```python
from build123d import *

# Parameters (mm, degrees)
ESQUISSE1_W             = 32
ESQUISSE1_H             = 8
BOSS_EXTRU_1_DEPTH      = 2
BOSS_EXTRU_2_DEPTH      = 2
ESQUISSE3_R             = 1.9999999999999996
ESQUISSE3_R_2           = 2.000000000000003
ESQUISSE3_R_3           = 1.9999999999999991
BOSS_EXTRU_3_DEPTH      = 2
ESQUISSE4_R             = 1.2499999999999991
ESQUISSE4_R_2           = 1.250000000000001
ESQUISSE4_R_3           = 1.2500000000000013
ENL_V_MAT_EXTRU_1_DEPTH = 2
CONG_1_R                = 1.5


with BuildPart() as part:
    # Esquisse1 → Boss.-Extru.1 (new body)
    with BuildSketch(Plane(origin=(0, 0, 0), x_dir=(1, 0, 0), z_dir=(0, 1, 0))):
        with Locations((16, 4)):
            Rectangle(ESQUISSE1_W, ESQUISSE1_H)
    extrude(amount=BOSS_EXTRU_1_DEPTH)

    # Esquisse2 → Boss.-Extru.2 (add)
    with BuildSketch(Plane(origin=(0, 2, 0), x_dir=(1, 0, 0), z_dir=(0, 1, 0))):
        Polygon((8.000000000000002, 4.5e-16), (24, 2.41e-15), (24.000000000000004, -17), (8.000000000000004, -17), align=None)
    extrude(amount=-BOSS_EXTRU_2_DEPTH)

    # Esquisse3 → Boss.-Extru.3 (add)
    with BuildSketch(Plane(origin=(0, 2, 0), x_dir=(1, 0, 0), z_dir=(0, 1, 0))):
        with Locations((8.000000000000002, 0)):
            Circle(ESQUISSE3_R)
        with Locations((24, 2.41e-15)):
            Circle(ESQUISSE3_R_2)
        with Locations((16.000000000000004, -17)):
            Circle(ESQUISSE3_R_3)
    extrude(amount=-BOSS_EXTRU_3_DEPTH)

    # Esquisse4 → Enlèv. mat.-Extru.1 (cut)
    with BuildSketch(Plane(origin=(0, 2, 0), x_dir=(1, 0, 0), z_dir=(0, 1, 0))):
        with Locations(Location((8.000000000000002, 0, 0), (0, 0, 270))):
            Circle(ESQUISSE4_R)
        with Locations(Location((24, 2.41e-15, 0), (0, 0, 270))):
            Circle(ESQUISSE4_R_2)
        with Locations(Location((16.000000000000004, -17, 0), (0, 0, 270))):
            Circle(ESQUISSE4_R_3)
    extrude(amount=-ENL_V_MAT_EXTRU_1_DEPTH, mode=Mode.SUBTRACT)

    # Congé1
    cong_1_edges = [part.edges().sort_by_distance(p)[0] for p in [
        (32, 2, -4),
        (16, 2, -8),
        (11.000000000000004, 2, 17),
        (24.000000000000004, 2, 9.500000000000002),
        (8.000000000000004, 2, 9.5),
        (29, 2, 0),
        (0, 2, -4),
        (21.000000000000004, 2, 17),
        (3.000000000000001, 2, 0),
    ]]
    fillet(cong_1_edges, radius=CONG_1_R)


solid = part.part
```
The model under review builds one solid part; all positions refer to its coordinate system, in mm. Round coordinates to 2 decimals unless told otherwise and drop trailing zeros. Write each loop counter-clockwise with the first axis right and the second up, starting at its lowest first coordinate (ties: lowest second). Pieces come first, ordered by that corner, then holes. Notation, with made-up numbers: (-11, -14.75) - (41, -14.75) arc R28 ccw to (41, 18.25) - close; hole circle Ø8 at (68.25, -18). An arc over 180 degrees is marked (long way). Use one line per item in the form item = value.
Q1. For line 1 (X direction, y = 1.5, z = 0); line 2 (X direction, y = 1.05, z = 17); line 3 (Z direction, x = 25, y = 0.8), list the stretches that pass through material, from the lowest coordinate up. Write a range as [from, to].
Answer key:
line_1 = [6, 6.75], [9.25, 22.75], [25.25, 26]
line_2 = [14, 14.75], [17.25, 18]
line_3 = [-7.97, -0.75], [0.75, 1.73]
Q2. Insertion check: pin 1 Ø0.6 at (x, y) = (3.5, 0) entering from +Z; pin 2 Ø0.6 at (x, y) = (12, 0) entering from +Z; pin 3 Ø1 at (y, z) = (1, 14.5) entering from -X. Each pin has a flat end and moves straight along its axis. Give the tip position at first contact, or say it passes through.
Answer key:
pin_1 = 0
pin_2 = 17
pin_3 = 8
Q3. Draft analysis for pull direction X (two halves, no side actions). For faces 1 (the cylindrical face through (28.71, 1.55, -0.43)), 2 (the cylindrical face through (22.891, 1.014, 0.577)), 3 (the cylindrical face through (31.57, 1.55, -4.06)), state which applies: +X half, -X half, draft (parallel to the pull), parting line (faces both ways), or undercut.
Answer key:
face_1 = draft
face_2 = undercut
face_3 = +X half
Q4. Consider section A-A (x = 16). State the section outline as (y, z) points.
Answer key:
outline = (0, -8) - (0.5, -8) arc R1.5 ccw to (2, -6.5) - (2, 15.75) - (0, 15.75) - close; (0, 18.25) - (2, 18.25) - (2, 19) - (0, 19) - close
Q5. Consider section D-D (z = -4.5). State the section outline as (x, y) points, and give its area (3 significant figures).
Answer key:
outline = (0, 0) - (32, 0) - (32, 0.5) arc R1.5 ccw to (30.5, 2) - (1.5, 2) arc R1.5 ccw to (0, 0.5) - close
area = 63.0 mm2
Q6. Consider section C-C (x = 27.5). State the section outline as (y, z) points, and give its area (3 significant figures).
Answer key:
outline = (0, -8) - (0.5, -8) arc R1.5 ccw to (2, -6.5) - (2, -1.5) arc R1.5 ccw to (0.5, 0) - (0, 0) - close
area = 15.0 mm2
